Autodesk Inventor part; units mm, degrees
ref_plane "YZ Plane" through (0, 0, 0) normal (1, 0, 0) x (0, 1, 0)
ref_plane "XZ Plane" through (0, 0, 0) normal (0, 1, 0) x (-1, 0, 0)
ref_plane "XY Plane" through (0, 0, 0) normal (0, 0, 1) x (1, 0, 0)
sketch "Sketch1" plane through (0, 0, 0) normal (0, 1, 0) x (-1, 0, 0)
  line L0 (6.35, 0) -> (146.05, 0)
  line L1 (152.4, -6.35) -> (152.4, -146.05)
  line L2 (146.05, -152.4) -> (6.35, -152.4)
  line L3 (0, -146.05) -> (0, -6.35)
  arc A0 (146.05, -152.4) -> (152.4, -146.05) centre (146.05, -146.05) ccw
  arc A1 (152.4, -6.35) -> (146.05, 0) centre (146.05, -6.35) ccw
  arc A2 (0, -146.05) -> (6.35, -152.4) centre (6.35, -146.05) ccw
  arc A3 (152.4, -6.35) -> (146.05, 0) centre (146.05, -6.35) ccw
  arc A4 (6.35, 0) -> (0, -6.35) centre (6.35, -6.35) ccw
  line L4 (147.6248, -146.05) -> (147.6248, -6.35)
  arc A5 (147.6248, -6.35) -> (146.05, -4.7752) centre (146.05, -6.35) ccw
  line L5 (146.05, -4.7752) -> (6.35, -4.7752)
  arc A6 (6.35, -4.7752) -> (4.7752, -6.35) centre (6.35, -6.35) ccw
  line L6 (4.7752, -6.35) -> (4.7752, -146.05)
  arc A7 (4.7752, -146.05) -> (6.35, -147.6248) centre (6.35, -146.05) ccw
  line L7 (6.35, -147.6248) -> (146.05, -147.6248)
  arc A8 (146.05, -147.6248) -> (147.6248, -146.05) centre (146.05, -146.05) ccw
  point P0 (0, 0)
  point P1 (152.4, -152.4)
  point P2 (152.4, 0)
  point P3 (0, -152.4)
  dimension "d0" = 152.4
  dimension "d1" = 152.4
  dimension "d2" = 6.35
  dimension "d3" = 6.35
  dimension "d4" = 6.35
  dimension "d5" = 4.7752
extrude "Extrusion1" add sketch "Sketch1" along normal blind 1828.8
properties part number "21015-22-1-3- 6X6 Stanchion" material "Steel, Carbon"
Verification items for the finished model (mm, model axes). A direction names the side the tool comes from. Round coordinates to 2 decimals unless told otherwise and drop trailing zeros. Write each loop counter-clockwise with the first axis right and the second up, starting at its lowest first coordinate (ties: lowest second). Pieces come first, ordered by that corner, then holes. Notation, with made-up numbers: (12.25, -23) - (33.25, -23) arc R14 ccw to (33.25, 1) - close; hole circle Ø1 at (-30, 66.5). An arc over 180 degrees is marked (long way). Answer as a JSON object with one key per item and string values. Group by question number.
Q1. Section check C-C, the plane x = -81.5. Enter the section's corners in (y, z), plus the area to 3 significant figures.
Q2. Section check A-A, the plane y = 1700. Enter the section's corners in (x, z), plus the area to 3 significant figures.
Q3. Tool access check on faces 1 (the flat face through (-77, 902, -4.775)), 2 (the flat face through (-70, 1828.8, -149)). Record the directions out of +Z, -Z, +X, -X, +Y, -Y that give a thin tool (end or side, any length) a straight path to the whole face; none if there is none.
Q4. Mould release check, pull along Z, two halves, no side actions. Record for faces 3 (the flat face through (-4.775, 902, -75)), 4 (the flat face through (-75, 902, 0)), 5 (the flat face through (-147.625, 902, -77)), 6 (the flat face through (-70, 0, -149)): released by +Z, released by -Z, zero draft, split by the parting line, or undercut.
Q5. Section check B-B, the plane z = -66. Enter the section's corners in (x, y).
Q6. Thickness scan on line 1 (X direction, y = 1443, z = -82.5). Record the ranges inside material, lowest first.
Found:
{
 "1": {"outline": "(0, -152.4) - (1828.8, -152.4) - (1828.8, -147.62) - (0, -147.62) - close; (0, -4.78) - (1828.8, -4.78) - (1828.8, 0) - (0, 0) - close", "area": "17,500 mm^2"},
 "2": {"outline": "(-152.4, -146.05) arc R6.35 ccw to (-146.05, -152.4) - (-6.35, -152.4) arc R6.35 ccw to (0, -146.05) - (0, -6.35) arc R6.35 ccw to (-6.35, 0) - (-146.05, 0) arc R6.35 ccw to (-152.4, -6.35) - close; hole (-147.62, -146.05) arc R1.57 ccw to (-146.05, -147.62) - (-6.35, -147.62) arc R1.57 ccw to (-4.78, -146.05) - (-4.78, -6.35) arc R1.57 ccw to (-6.35, -4.78) - (-146.05, -4.78) arc R1.57 ccw to (-147.62, -6.35) - close", "area": "2,790 mm^2"},
 "3": {"face 1": "+Y, -Y", "face 2": "+Z, -Z, +X, -X, +Y"},
 "4": {"face 3": "undercut", "face 4": "released by +Z", "face 5": "undercut", "face 6": "zero draft"},
 "5": {"outline": "(-152.4, 0) - (-147.62, 0) - (-147.62, 1828.8) - (-152.4, 1828.8) - close; (-4.78, 0) - (0, 0) - (0, 1828.8) - (-4.78, 1828.8) - close"},
 "6": {"line 1": "x = -152.4 to -147.62, -4.78 to 0"}
}
